Autodesk Inventor part; units mm, degrees
ref_plane "YZ Plane" through (0, 0, 0) normal (1, 0, 0) x (0, 1, 0)
ref_plane "XZ Plane" through (0, 0, 0) normal (0, 1, 0) x (-1, 0, 0)
ref_plane "XY Plane" through (0, 0, 0) normal (0, 0, 1) x (1, 0, 0)
sketch "Sketch1" plane through (0, 0, 0) normal (0, 1, 0) x (-1, 0, 0)
  line L0 (0, 0) -> (0, -167.039) construction
  line L1 (-3, 0) -> (-3, -167.039)
  line L2 (3, -167.039) -> (3, 0)
  arc A0 (3, 0) -> (-3, 0) centre (0, 0) ccw
  arc A1 (-3, -167.039) -> (3, -167.039) centre (0, -167.039) ccw
  circle A2 centre (0, 0) radius 1.5
  circle A3 centre (0, -167.039) radius 1.5
  circle A4 centre (0, -57.227) radius 1.5
  arc A5 (3, -167.039) -> (3, -57.227) centre (-393.2137, -112.133) ccw
  arc A6 (-3, -167.039) -> (-3, -57.227) centre (-399.2137, -112.133) ccw
  arc A7 (-3, -55) -> (-3, -15) centre (-48.8258, -35) ccw
  arc A8 (3, -55) -> (3, -15) centre (-42.8258, -35) ccw
  point P0 (0, -83.5195)
  dimension "d0" = 167.039
  dimension "d1" = 6
  dimension "d2" = 3
  dimension "d3" = 3
  dimension "d10" = 3
  dimension "d11" = 57.227
  dimension "d12" = 400
  dimension "d13" = 400
  dimension "d16" = 15
  dimension "d17" = 55
  dimension "d18" = 50
  dimension "d19" = 50
extrude "Extrusion1" add sketch "Sketch1" along normal blind 8 contours A0 L2 A1 A6 L1 A7 | A8 L2 | A5 L2
fillet "Fillet1" radius 10 6 edges at (-3, 4, -15) (3, 4, -15) (-3, 4, -55) (3, 4, -55) (-3, 4, -57.227) (3, 4, -57.227)
sketch "Sketch2" plane through (0, 0, 0) normal (0, -1, 0) x (1, 0, 0)
  circle A0 centre (0, -57.227) radius 1.5
  circle A1 centre (0, -167.039) radius 1.5
  circle A2 centre (0, 0) radius 1.5
  arc A3 (2.8635, -58.2209) -> (2.2666, -53.2276) centre (-7.0452, -56.8731) ccw
  arc A4 (2.3043, -16.6764) -> (2.2666, -53.2276) centre (48.8258, -35) ccw
  arc A5 (2.3043, -16.6764) -> (3, -13.0117) centre (-7, -13.0117) ccw
  line L0 (3, 0) -> (3, -13.0117)
  arc A6 (3, 0) -> (-3, 0) centre (0, 0) ccw
  line L1 (-3, -13.0117) -> (-3, 0)
  arc A7 (-3.6957, -16.6764) -> (-3, -13.0117) centre (-13, -13.0117) ccw
  arc A8 (-3.6957, -16.6764) -> (-3.7334, -53.2276) centre (42.8258, -35) ccw
  arc A9 (-3.1365, -58.2209) -> (-3.7334, -53.2276) centre (-13.0452, -56.8731) ccw
  arc A10 (-3.1365, -58.2209) -> (-3, -167.039) centre (393.2137, -112.133) ccw
  arc A11 (-3, -167.039) -> (3, -167.039) centre (0, -167.039) ccw
  arc A12 (2.8635, -58.2209) -> (3, -167.039) centre (399.2137, -112.133) ccw
Design review of the part built by this model. Coordinates are the model's own, in mm. A direction names the side the tool comes from. Give positions to 0.01 mm unless a question says otherwise; leave off trailing zeros. Loops run counter-clockwise (first coordinate to the right, second up) from the corner with the lowest first, then second, coordinate; pieces in that order, holes last. Notation, with made-up numbers: (30, 76) -> (66, 76) arc R26 ccw to (66, 105) -> close; hole circle Ø7 at (-18, 52.25). An arc over 180 degrees is marked (long way). Write each question's results on one line, items separated by ' | '.
Q1. Take a section at A-A, the plane y = 6.25. Give the number of separate pieces and of enclosed holes in the cut face, plus the area to 3 significant figures.
Reply:
separate pieces: 1 | enclosed holes: 3 | area: 1,010 mm²
Q2. Take a section at B-B, the plane z = -30.5. Write out the cut boundary in (x, y).
Reply:
outline: (-6.97, 0) -> (-0.97, 0) -> (-0.97, 8) -> (-6.97, 8) -> close
Q3. For pin 1 Ø1.8 at (x, z) = (0, -167.039) entering from -Y; pin 2 Ø4 at (y, z) = (2.5, -6) entering from -X; pin 3 Ø1 at (y, z) = (5, -95.5) entering from +X; pin 4 Ø1 at (y, z) = (3, -27.5) entering from -X, all flat-tipped, find the tip position at first contact; note any pin that passes through.
Reply:
pin 1: passes through | pin 2: stops at x = -3 | pin 3: stops at x = -0.42 | pin 4: stops at x = -6.68
Q4. The part is to be moulded in two halves that separate along Z. For faces 1 (the face through (0.195, 3.944, -58.714)), 2 (the face through (-0.07, 3.94, -170.04)), 3 (the face through (-3, 4, -7)), 4 (the face through (-0.786, 3.944, -111.87)), say which applies: +Z half, -Z half, draft (parallel to the pull), parting line (faces both ways), or undercut.
Reply:
face 1: undercut | face 2: -Z half | face 3: draft | face 4: undercut
Q5. Machinability: for faces 5 (the face through (0, 4, 3)), 6 (the face through (2.83, 4.06, -14.85)), which of the approach directions +Z, -Z, +X, -X, +Y, -Y give a long, thin tool a straight path to every point of the face, cutting with its end or side? Answer none if there is none.
Reply:
face 5: +Z, +Y, -Y | face 6: +X, +Y, -Y
Q6. Wall thickness on L1, parallel to X at y = 5.5, z = -109; L2, parallel to X at y = 1.25, z = -84.5; L3, parallel to Z at x = -2, y = 4.5: over which ranges is each line inside the solid? List them lowest first.
Reply:
L1: x = -6.77 to -0.77 | L2: x = -5.83 to 0.17 | L3: z = -169.28 to 2.24
